from build123d import *

# Parameters (mm, degrees)
EXTRUDE_THIN1_DEPTH = 24
FILLET1_R           = 1
FILLET2_R           = 0.2


with BuildPart() as part:
    # Sketch1 → Extrude-Thin1 (new body)
    with BuildSketch(Plane.XY):
        Polygon((3.75, 8), (3.75, 7), (5, 2.8), (5, 1.8), (4, 1.8), (4, 0), (-4, 0), (-4, 1.8), (-5, 1.8), (-5, 2.8), (-3.75, 7), (-3.75, 8), (-3.35, 8), (-3.35, 6.941738969), (-4.6, 2.741738969), (-4.6, 2.2), (-3.6, 2.2), (-3.6, 0.4), (3.6, 0.4), (3.6, 2.2), (4.6, 2.2), (4.6, 2.741738969), (3.35, 6.941738969), (3.35, 8), align=None)
    extrude(amount=EXTRUDE_THIN1_DEPTH)

    # Fillet1
    fillet1_edges = [part.edges().sort_by_distance(p)[0] for p in [
        (4, 0, 12),
        (-4, 0, 12),
        (-3.6, 0.4, 12),
        (3.6, 0.4, 12),
    ]]
    fillet(fillet1_edges, radius=FILLET1_R)

    # Fillet2
    fillet2_edges = [part.edges().sort_by_distance(p)[0] for p in [
        (5, 2.8, 12),
        (5, 1.8, 12),
        (4, 1.8, 12),
        (-4, 1.8, 12),
        (-5, 1.8, 12),
        (-5, 2.8, 12),
        (-4.6, 2.741738969, 12),
        (-4.6, 2.2, 12),
        (-3.6, 2.2, 12),
        (3.6, 2.2, 12),
        (4.6, 2.2, 12),
        (4.6, 2.741738969, 12),
    ]]
    fillet(fillet2_edges, radius=FILLET2_R)


solid = part.part
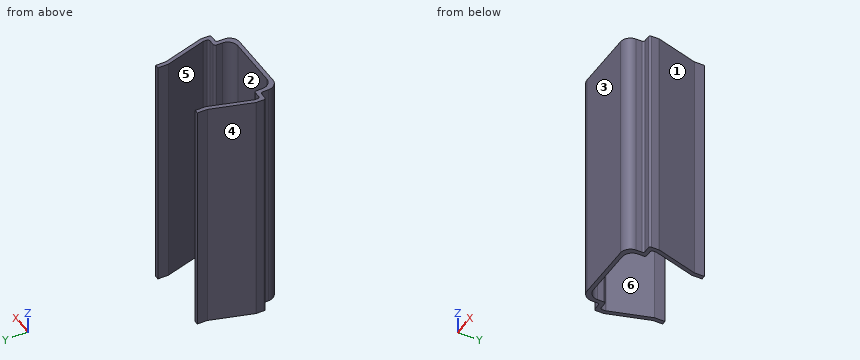
Verification items for the finished model (mm, model axes). Face numbers are marked on the shaded views. A direction names the side the tool comes from. Coordinates: 2 decimals unless noted, no trailing zeros. Order: outer loops, then holes, each group sorted by start corner. A loop starts at its lowest first (then second) coordinate and runs counter-clockwise, first axis right, second up. Notation, with made-up numbers: M -3.5,12 L 4.5,12 A19 ccw 4.5,33 Z; hole C -17,56.25 d10. An arc over 180 degrees is marked long. One line per item, written item: value. Start each with the question number.
Item 1: Scan lines: probe 1 along X at (y, z) = (2, 20); probe 2 along Y at (x, z) = (1, 21.25); probe 3 along X at (y, z) = (1, 3.5). Record each from-to range of solid material in increasing order.
Item 2: Gauge pin test, flat ends, axial feed: pin 1 (0.5 mm diameter, centred on y = 7.5, z = 17.5, fed in from -X); pin 2 (1 mm diameter, centred on x = 3, z = 13, fed in from +Y); pin 3 (0.8 mm diameter, centred on y = 7.5, z = 16.5, fed in from +X); pin 4 (3 mm diameter, centred on y = 6, z = 7.5, fed in from +X). Record the tip position at first contact, or that the pin passes through.
Item 3: Access from +Z, -Z, +X, -X, +Y, -Y to the whole of each face (thin tool, end or side, straight path). Record for the marked faces 1 and 2.
Item 4: Sectioned sample at A-A (y = 5.5). Enter the section's corners in (x, z), then the cut area to 3 significant figures.
Item 5: Mould release check, pull along X, two halves, no side actions. Record for the marked faces 3, 4, 5 and 6: released by +X, released by -X, zero draft, split by the parting line, or undercut.
Conclusion:
1. probe 1: x = -5 to -3.6, 3.6 to 5
1. probe 2: y = 0 to 0.4
1. probe 3: x = -4 to -3.52, 3.52 to 4
2. pin 1: stops at x = -3.75
2. pin 2: stops at y = 8
2. pin 3: stops at x = 3.75
2. pin 4: stops at x = 4.49
3. face 1: +Z, -Z, +X, +Y
3. face 2: +Z, -Z, +Y
4. outline: M -4.2,0 L -3.78,0 L -3.78,24 L -4.2,24 Z; M 3.78,0 L 4.2,0 L 4.2,24 L 3.78,24 Z
4. area: 20.0 mm^2
5. face 3: zero draft
5. face 4: released by -X
5. face 5: undercut
5. face 6: undercut
